Check sheet for the modelled part. Datum: model origin and axes. Units: mm. Face numbers are marked on the shaded views. A direction names the side the tool comes from. Round coordinates to 2 decimals unless told otherwise and drop trailing zeros. Order: outer loops, then holes, each group sorted by start corner. A loop starts at its lowest first (then second) coordinate and runs counter-clockwise, first axis right, second up.
Q1. Cross-section at C-C on x = -42.5. Record the cut outline in (y, z), then the cut area to 3 significant figures.
Q2. Cross-section at B-B on z = -8. Record the cut outline in (x, y).
Q3. Set-up check for the marked faces 5, 6 and 7: record each of +Z, -Z, +X, -X, +Y, -Y from which the full face is reachable in a straight line by a thin tool's end or side.
Q4. Cross-section at D-D on x = -12. Record the cut outline in (y, z), then the cut area to 3 significant figures.
Q5. Cross-section at A-A on y = 50. Give the number of separate pieces and of enclosed holes in the cut face, then the cut area to 3 significant figures.
Q6. Mould release check, pull along X, two halves, no side actions. Record for the marked faces 1, 2, 3 and 4: +X half, -X half, draft (parallel to the pull), parting line (faces both ways), or undercut.
Q7. Scan lines: probe 1 along X at (y, z) = (19.5, -0.5); probe 2 along X at (y, z) = (38, -7); probe 3 along X at (y, z) = (50, 17). Record each from-to range of solid material in increasing order.
Q8. Depth check by flat-ended pin: P1, Ø3, axis at x = -2, y = 32.5, coming from the +Z side; P2, Ø5, axis at x = 11, z = 9, coming from the +Y side; P3, Ø1.5, axis at y = 38, z = 18, coming from the +X side; P4, Ø1, axis at x = -22, y = 16, coming from the +Z side. Enter the tip coordinate at first touch or a pass-through.
from build123d import *

# Parameters (mm, degrees)
BOSS_EXTRU_1_DEPTH           = 60
CONG_3_R                     = 1
ENL_V_MAT_EXTRU_1_DEPTH      = 60
ENL_V_MAT_EXTRU_2_DEPTH      = 90.469797558
ENL_V_MAT_EXTRU_2_DEPTH_BACK = 60


with BuildPart() as part:
    # Esquisse1 → Boss.-Extru.1 (new body)
    with BuildSketch(Plane(origin=(0, 0, 0), x_dir=(1, 0, 0), z_dir=(0, 1, 0))):
        Polygon((-21.960784314, -19.516817925), (-21.960784314, 20.483182075), (16.039215686, 20.483182075), (12.222833137, -19.516817925), (15.222833137, -19.516817925), (19.325444377, 23.483182075), (-24.960784314, 23.483182075), (-24.960784314, -16.516817925), (-49.960784314, -16.516817925), (-49.960784314, 23.483182075), (-52.960784314, 23.483182075), (-52.960784314, -19.516817925), align=None)
    extrude(amount=BOSS_EXTRU_1_DEPTH)

    # Cong_3
    cong_3_edges = [part.edges().sort_by_distance(p)[0] for p in [
        (-52.960784314, 30, 19.516817925),
        (-52.960784314, 30, -23.483182075),
        (-49.960784314, 30, -23.483182075),
        (-49.960784314, 30, 16.516817925),
        (-24.960784314, 30, 16.516817925),
        (-24.960784314, 30, -23.483182075),
        (19.325444377, 30, -23.483182075),
        (15.222833137, 30, 19.516817925),
        (12.222833137, 30, 19.516817925),
        (16.039215686, 30, -20.483182075),
        (-21.960784314, 30, -20.483182075),
        (-21.960784314, 30, 19.516817925),
    ]]
    fillet(cong_3_edges, radius=CONG_3_R)

    # Esquisse2 → Enl_v. mat.-Extru.1 (cut)
    with BuildSketch(Plane(origin=(0, 0, 16.516817925), x_dir=(-1, 0, 0), z_dir=(0, 0, -1))):
        with BuildLine():
            Line((41.358290676, 7.5), (41.358290676, 52.5))
            ThreePointArc((41.358290676, 52.5), (42.711362899, 53.853072223), (44.064435122, 52.5))
            Line((44.064435122, 52.5), (44.064435122, 7.5))
            ThreePointArc((44.064435122, 7.5), (42.711362899, 6.146927777), (41.358290676, 7.5))
        make_face()
    extrude(amount=-ENL_V_MAT_EXTRU_1_DEPTH, mode=Mode.SUBTRACT)

    # Esquisse2_4 → Enl_v. mat.-Extru.2 (cut, two sides: drawn at the far end of the back side and taken through both)
    with BuildSketch(Plane(origin=(0, 0, 16.516817925), x_dir=(-1, 0, 0), z_dir=(0, 0, -1)).offset(-ENL_V_MAT_EXTRU_2_DEPTH_BACK)):
        with BuildLine():
            Line((28.538681886, 7.5), (28.538681886, 52.5))
            ThreePointArc((28.538681886, 52.5), (30.038681886, 54), (31.538681886, 52.5))
            Line((31.538681886, 52.5), (31.538681886, 7.5))
            ThreePointArc((31.538681886, 7.5), (30.038681886, 6), (28.538681886, 7.5))
        make_face()
    extrude(amount=ENL_V_MAT_EXTRU_2_DEPTH + ENL_V_MAT_EXTRU_2_DEPTH_BACK, mode=Mode.SUBTRACT)


solid = part.part
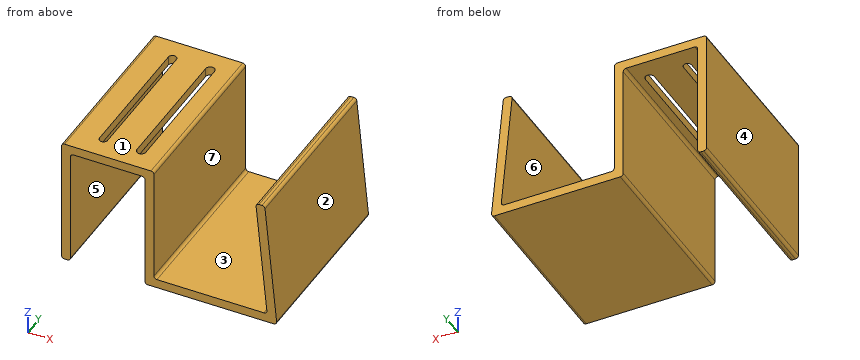
Results found:
1. outline: (0, 16.52) - (6.16, 16.52) - (6.16, 19.52) - (0, 19.52) - close; (53.84, 16.52) - (60, 16.52) - (60, 19.52) - (53.84, 19.52) - close
1. area: 37.0 mm2
2. outline: (-52.96, 0) - (-49.96, 0) - (-49.96, 60) - (-52.96, 60) - close; (-24.96, 0) - (-21.96, 0) - (-21.96, 60) - (-24.96, 60) - close; (14.85, 0) - (17.85, 0) - (17.85, 60) - (14.85, 60) - close
3. face 5: -Z, +Y, -Y
3. face 6: +Y, -Y
3. face 7: +Z, +Y, -Y
4. outline: (0, -23.48) - (60, -23.48) - (60, -20.48) - (0, -20.48) - close
4. area: 180 mm2
5. separate pieces: 3
5. enclosed holes: 0
5. area: 558 mm2
6. face 1: draft
6. face 2: +X half
6. face 3: undercut
6. face 4: -X half
7. probe 1: x = -52.96 to -49.96, -24.96 to -21.96, 14.13 to 17.13
7. probe 2: x = -52.96 to -49.96, -24.96 to -21.96, 14.75 to 17.75
7. probe 3: x = -52.96 to -44.06, -41.36 to -31.54, -28.54 to -21.96, 12.46 to 15.46
8. P1: stops at z = -20.48
8. P2: stops at y = 60
8. P3: stops at x = 15.44
8. P4: stops at z = 19.4
